CAD build for the part. Positions are in the model's coordinates, mm. Face numbers are marked on the shaded views. A direction names the side the tool comes from. Give positions to 0.01 mm unless a question says otherwise; leave off trailing zeros. Order: outer loops, then holes, each group sorted by start corner. A loop starts at its lowest first (then second) coordinate and runs counter-clockwise, first axis right, second up. Notation, with made-up numbers: M 69,57 L 103,57 A34 ccw 103,93 Z; hole C 68,-27 d1. An arc over 180 degrees is marked long. Put each result on its own line as item: value. Start each with the question number.
1) Cut at C-C (x = -0.5). Write the cut outline in (y, z), and give its area (4 significant figures).
2) Two-plate mould, pull along Z, no slides. Class the marked faces 6, 7 and 8: released by +Z, released by -Z, zero draft, split by the parting line, or undercut.
3) Tool access for the marked faces 1, 2, 3, 4 and 5: list every direction of +Z, -Z, +X, -X, +Y, -Y with a clear straight run to the whole face (end or side of a thin tool).
4) Cut at B-B (z = -12). Write the cut outline in (x, y), and give its area (3 significant figures).
5) Cut at D-D (z = -5.5). Write the cut outline in (x, y).
6) Drill centre lines: line 1 (X direction, y = 0.95, z = -12); line 2 (Z direction, x = -0.5, y = 3.5); line 3 (Y direction, x = -6.5, z = 10.5). Where is each one in solid material? Low to high. Write a range as [from, to].
7) Pin check, flat tips, straight feed: pin 1 (4 mm diameter, centred on y = 4, z = -15, fed in from -X); pin 2 (12 mm diameter, centred on x = 5, z = 5.5, fed in from +Y); pin 3 (2.5 mm diameter, centred on y = 5, z = -4, fed in from -X). Stop position of each tip, or through.
8) Cut at A-A (y = 4). Write the cut outline in (x, z), and give its area (3 significant figures).
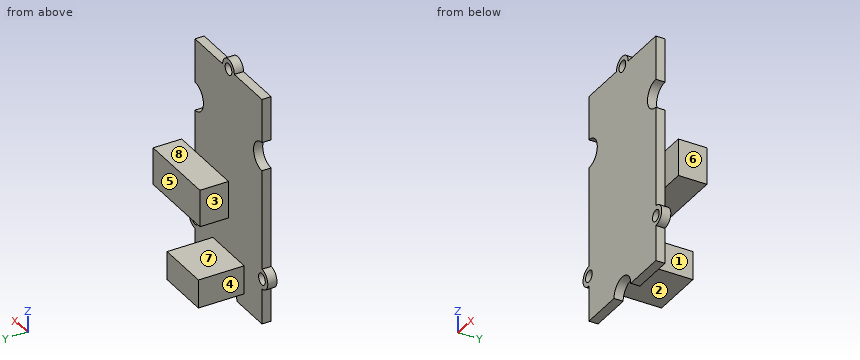
```python
from build123d import *

# Parameters (mm, degrees)
SKETCH1_R                 = 1
PCB_DEPTH                 = 1.6
SKETCH2_W                 = 10
SKETCH2_H                 = 6.5
SKETCH2_W_2               = 4
ELECTRODE_CONNECTOR_DEPTH = 5
SKETCH2_3_W               = 4.684517913
SKETCH2_3_H               = 5
CONTROL_CONNECTOR_DEPTH   = 8


with BuildPart() as part:
    # Sketch1 → PCB (new body)
    with BuildSketch(Plane(origin=(0, 0, 0), x_dir=(1, 0, 0), z_dir=(0, 1, 0))):
        with BuildLine():
            ThreePointArc((-1.75, -20), (0, -21.75), (1.75, -20))
            Line((1.75, -20), (10, -20))
            Line((10, -20), (10, -12.3))
            ThreePointArc((10, -12.3), (7.5, -9.8), (10, -7.3))
            Line((10, -7.3), (10, 10.25))
            ThreePointArc((10, 10.25), (11.75, 12), (10, 13.75))
            Line((10, 13.75), (10, 20))
            Line((10, 20), (2.5, 20))
            ThreePointArc((2.5, 20), (0, 17.5), (-2.5, 20))
            Line((-2.5, 20), (-10, 20))
            Line((-10, 20), (-10, 13.75))
            ThreePointArc((-10, 13.75), (-11.75, 12), (-10, 10.25))
            Line((-10, 10.25), (-10, -7.3))
            ThreePointArc((-10, -7.3), (-7.5, -9.8), (-10, -12.3))
            Line((-10, -12.3), (-10, -20))
            Line((-10, -20), (-1.75, -20))
        make_face()
        with Locations(Location((0, -20, 0), (0, 0, 270))):
            Circle(SKETCH1_R, mode=Mode.SUBTRACT)
        with Locations(Location((10, 12, 0), (0, 0, 270))):
            Circle(SKETCH1_R, mode=Mode.SUBTRACT)
        with Locations(Location((-10, 12, 0), (0, 0, 270))):
            Circle(SKETCH1_R, mode=Mode.SUBTRACT)
    extrude(amount=PCB_DEPTH)

    # Sketch2 → Electrode_connector (add)
    with BuildSketch(Plane(origin=(0, 1.6, 0), x_dir=(1, 0, 0), z_dir=(0, 1, 0))):
        with Locations((5, 3.25)):
            Rectangle(SKETCH2_W, SKETCH2_H)
        with Locations((12, 3.25)):
            Rectangle(SKETCH2_W_2, SKETCH2_H)
    extrude(amount=ELECTRODE_CONNECTOR_DEPTH)

    # Sketch2_3 → Control_connector (add)
    with BuildSketch(Plane(origin=(0, 1.6, 0), x_dir=(1, 0, 0), z_dir=(0, 1, 0))):
        with Locations((-2.342258957, 15)):
            Rectangle(SKETCH2_3_W, SKETCH2_3_H)
        with Locations((2.342258957, 15)):
            Rectangle(SKETCH2_3_W, SKETCH2_3_H)
    extrude(amount=CONTROL_CONNECTOR_DEPTH)


solid = part.part
```
Solution:
1. outline: M 0,-17.55 L 1.6,-17.55 L 1.6,-17.5 L 9.6,-17.5 L 9.6,-12.5 L 1.6,-12.5 L 1.6,19.13 L 0,19.13 Z; M 0,20.87 L 1.6,20.87 L 1.6,21.68 L 0,21.68 Z
1. area: 100.0 mm²
2. face 6: zero draft
2. face 7: undercut
2. face 8: released by +Z
3. face 1: -Z, +X, +Y
3. face 2: -Z, +X, -X, +Y
3. face 3: +Z, -X, +Y
3. face 4: +Z, -Z, -X, +Y
3. face 5: +Z, +X, -X, +Y
4. outline: M -11.75,0 L -11,0 L -11,1.6 L -11.75,1.6 Z; M -9,0 L 9,0 L 9,1.6 L -9,1.6 Z; M 11,0 L 11.75,0 L 11.75,1.6 L 11,1.6 Z
4. area: 31.2 mm²
5. outline: M -10,0 L 10,0 L 10,1.6 L 14,1.6 L 14,6.6 L 0,6.6 L 0,1.6 L -10,1.6 Z
6. line 1: [-11.75, -11], [-9, 9], [11, 11.75]
6. line 2: [-17.5, -12.5]
6. line 3: [0, 1.6]
7. pin 1: x = -4.68
7. pin 2: y = 6.6
7. pin 3: x = 0
8. outline: M -4.68,-17.5 L 4.68,-17.5 L 4.68,-12.5 L -4.68,-12.5 Z; M 0,-6.5 L 14,-6.5 L 14,0 L 0,0 Z
8. area: 138 mm²
